Here's how the part is built. I have some questions about the finished solid (model axes, mm). A direction names the side the tool comes from. Round coordinates to 2 decimals unless told otherwise and drop trailing zeros. Write each loop counter-clockwise with the first axis right and the second up, starting at its lowest first coordinate (ties: lowest second). Pieces come first, ordered by that corner, then holes. Notation, with made-up numbers: M 5.5,-1.5 L 32.5,-1.5 A27 cw 32.5,35.5 Z; hole C 1.5,61.5 d4. An arc over 180 degrees is marked long. Write item = value, one per line. Start each with the question number.
(1) If we mould it in two halves opening along X, with no side actions, what happens to faces 4 (the flat face through (-2.625, 0, 1)), 5 (the cylindrical face through (-0.35, 0.29, 1.67)), 6 (the flat face through (-1, 0, 1.92))? For each: released by +X, released by -X, zero draft, split by the parting line, or undercut.
(2) I want a section at A-A (y = 0). List the corners of the cut face in (x, z) for me (3 decimals), and give its area (3 significant figures).
(3) Will this pin go through, and if not, where does the flat tip stop? pin 1 Ø2 at (x, z) = (0.5, -2) entering from +Y (3 decimals).
(4) I want a section at B-B (z = -2.75). List the corners of the cut face in (x, y) for me (3 decimals).
(5) On a 3-axis mill with a long thin cutter (end or side, diameter ignored), from which of +Z, -Z, +X, -X, +Y, -Y can I reach the whole of each face in a straight line? I mean faces 1 (the flat face through (0, 1.25, 1)), 2 (the flat face through (0, 0, 0)), 3 (the cylindrical face through (2.19, 0.29, 1.67)). Say none if no direction works.
(6) I want a section at D-D (z = -3.5). List the corners of the cut face in (x, y) for me, and give its area (3 significant figures).
(7) I want a section at C-C (x = -1.27). List the corners of the cut face in (y, z) for me (3 decimals), and give its area (3 significant figures).
(8) I need wall thicknesses on line 1 along Z through (x, y) = (-0.05, -0.65); line 2 along X through (y, z) = (0.6, -1.75); line 3 along Z through (x, y) = (-2.2, 0). Which ranges of each line are inside material? Lowest first, please.
```python
from build123d import *

# Parameters (mm, degrees)
SKETCH_1_W          = 5.25
SKETCH_1_H          = 2.5
EXTRUDE_1_DEPTH     = 1.42
SKETCH_2_R          = 0.725
EXTRUDE_2_DEPTH     = 5
SKETCH_3_R          = 0.965
EXTRUDE_3_DEPTH     = 0.5
CUT_EXTRUDE_START   = -2.1
SKETCH_4_R          = 0.725
SKETCH_4_R_2        = 0.42
CUT_EXTRUDE_1_DEPTH = 2.1


with BuildPart() as part:
    # ｽｹｯﾁ1 → ﾎﾞｽ - 押し出し1 (new body)
    with BuildSketch(Plane.XY):
        Rectangle(SKETCH_1_W, SKETCH_1_H)
    extrude(amount=EXTRUDE_1_DEPTH)

    # ｽｹｯﾁ2 → ﾎﾞｽ - 押し出し2 (add)
    with BuildSketch(Plane(origin=(0, 0, 0), x_dir=(-1, 0, 0), z_dir=(0, 0, -1))):
        with Locations(Location((-1.27, 0, 0), (0, 0, 180))):
            Circle(SKETCH_2_R)
        with Locations(Location((1.27, 0, 0), (0, 0, 180))):
            Circle(SKETCH_2_R)
    extrude(amount=EXTRUDE_2_DEPTH)

    # ｽｹｯﾁ3 → ﾎﾞｽ - 押し出し3 (add)
    with BuildSketch(Plane.XY.offset(1.42)):
        with Locations((-1.27, 0)):
            Circle(SKETCH_3_R)
        with Locations((1.27, 0)):
            Circle(SKETCH_3_R)
    extrude(amount=EXTRUDE_3_DEPTH)

    # ｽｹｯﾁ4 → ｶｯﾄ - 押し出し1 (cut)
    # profile 1 of 2: a face of its own
    with BuildSketch(Plane(origin=(0, 0, -5), x_dir=(-1, 0, 0), z_dir=(0, 0, -1)).offset(CUT_EXTRUDE_START)):
        with Locations(Location((-1.27, 0, 0), (0, 0, 180))):
            Circle(SKETCH_4_R)
        with Locations((-1.27, 0)):
            Circle(SKETCH_4_R_2, mode=Mode.SUBTRACT)
    # profile 2 of 2: a face of its own
    with BuildSketch(Plane(origin=(0, 0, -5), x_dir=(-1, 0, 0), z_dir=(0, 0, -1)).offset(CUT_EXTRUDE_START)):
        with Locations(Location((1.27, 0, 0), (0, 0, 180))):
            Circle(SKETCH_4_R)
        with Locations((1.27, 0)):
            Circle(SKETCH_4_R_2, mode=Mode.SUBTRACT)
    extrude(amount=CUT_EXTRUDE_1_DEPTH, mode=Mode.SUBTRACT)


solid = part.part
```
Returned:
q1.face_4 = released by -X
q1.face_5 = undercut
q1.face_6 = zero draft
q2.outline = M -2.625,0 L -1.995,0 L -1.995,-2.9 L -1.69,-2.9 L -1.69,-5 L -0.85,-5 L -0.85,-2.9 L -0.545,-2.9 L -0.545,0 L 0.545,0 L 0.545,-2.9 L 0.85,-2.9 L 0.85,-5 L 1.69,-5 L 1.69,-2.9 L 1.995,-2.9 L 1.995,0 L 2.625,0 L 2.625,1.42 L 2.235,1.42 L 2.235,1.92 L 0.305,1.92 L 0.305,1.42 L -0.305,1.42 L -0.305,1.92 L -2.235,1.92 L -2.235,1.42 L -2.625,1.42 Z
q2.area = 21.3 mm²
q3.pin_1 = 0.725
q4.outline = C -1.27,0 d1.45; C 1.27,0 d1.45
q5.face_1 = +Z, -Z, +X, -X, +Y
q5.face_2 = -Z
q5.face_3 = +Z
q6.outline = C -1.27,0 d0.84; C 1.27,0 d0.84
q6.area = 1.11 mm²
q7.outline = M -1.25,0 L -0.725,0 L -0.725,-2.9 L -0.42,-2.9 L -0.42,-5 L 0.42,-5 L 0.42,-2.9 L 0.725,-2.9 L 0.725,0 L 1.25,0 L 1.25,1.42 L 0.965,1.42 L 0.965,1.92 L -0.965,1.92 L -0.965,1.42 L -1.25,1.42 Z
q7.area = 10.5 mm²
q8.line_1 = 0 to 1.42
q8.line_2 = -1.68 to -0.86, 0.86 to 1.68
q8.line_3 = 0 to 1.92
